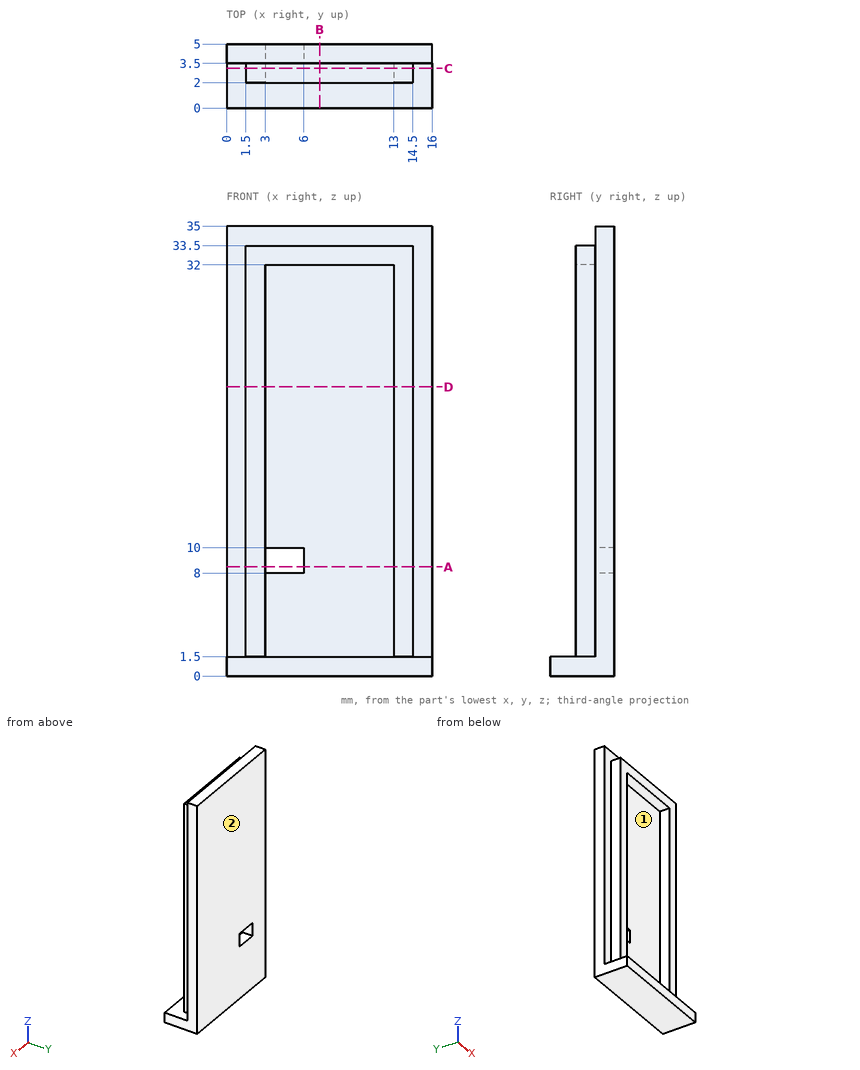
Job drawing, mm, ordinate dimensions from the low corner. One solid piece. Coordinates: 2 decimals unless noted, no trailing zeros. Order: outer loops, then holes, each group sorted by start corner. A loop starts at its lowest first (then second) coordinate and runs counter-clockwise, first axis right, second up. Notation, with made-up numbers: M 65.5,-2 L 105.5,-2 A21 ccw 105.5,28 Z; hole C -11,58.25 d4. An arc over 180 degrees is marked long. Answer as CSV lines item,"result".
(1) Wall check: line 1 along Z through (x, y) = (8, 2.15); line 2 along X through (y, z) = (3.65, 9.5); line 3 along X through (y, z) = (3.35, 15). Give the ranges that are in metal, low to high.
Geometry says:
line 1,"z = 0 to 1.5, 32 to 33.5"
line 2,"x = 0 to 3, 6 to 16"
line 3,"x = 1.5 to 3, 13 to 14.5"
(2) Band-saw the part on A-A, the plane z = 8.5. List the corners of the cut face in (x, y).
Geometry says:
outline,"M 0,3.5 L 1.5,3.5 L 1.5,2 L 3,2 L 3,5 L 0,5 Z; M 6,3.5 L 13,3.5 L 13,2 L 14.5,2 L 14.5,3.5 L 16,3.5 L 16,5 L 6,5 Z"
(3) Band-saw the part on D-D, the plane z = 22.5. List the corners of the cut face in (x, y).
Geometry says:
outline,"M 0,3.5 L 1.5,3.5 L 1.5,2 L 3,2 L 3,3.5 L 13,3.5 L 13,2 L 14.5,2 L 14.5,3.5 L 16,3.5 L 16,5 L 0,5 Z"
(4) Band-saw the part on C-C, the plane y = 3.1. List the corners of the cut face in (x, z).
Geometry says:
outline,"M 0,0 L 16,0 L 16,1.5 L 14.5,1.5 L 14.5,33.5 L 1.5,33.5 L 1.5,1.5 L 0,1.5 Z; hole M 3,1.5 L 13,1.5 L 13,32 L 3,32 Z"
(5) Flat gauge pins, fed straight in: pin 1 (3 mm diameter, centred on y = 1.5, z = 20, fed in from -X); pin 2 (5 mm diameter, centred on x = 9.5, z = 15.5, fed in from -Y); pin 3 (1 mm diameter, centred on x = 2, y = 2, fed in from -Z); pin 4 (1 mm diameter, centred on y = 2.5, z = 9.5, fed in from +X). Where does each tip first touch, or does it go through?
Geometry says:
pin 1,"stops at x = 1.5"
pin 2,"stops at y = 3.5"
pin 3,"stops at z = 0"
pin 4,"stops at x = 14.5"
(6) Pull direction X, two halves, no side cores. Call the marked faces 1 and 2: +X half, -X half, draft (parallel to the pull), parting line (faces both ways), or undercut.
Geometry says:
face 1,"undercut"
face 2,"draft"
(7) Band-saw the part on B-B, the plane x = 7.25. List the corners of the cut face in (y, z), then the cut area to 3 significant figures.
Geometry says:
outline,"M 0,0 L 5,0 L 5,35 L 3.5,35 L 3.5,33.5 L 2,33.5 L 2,32 L 3.5,32 L 3.5,1.5 L 0,1.5 Z"
area,"60.0 mm2"
